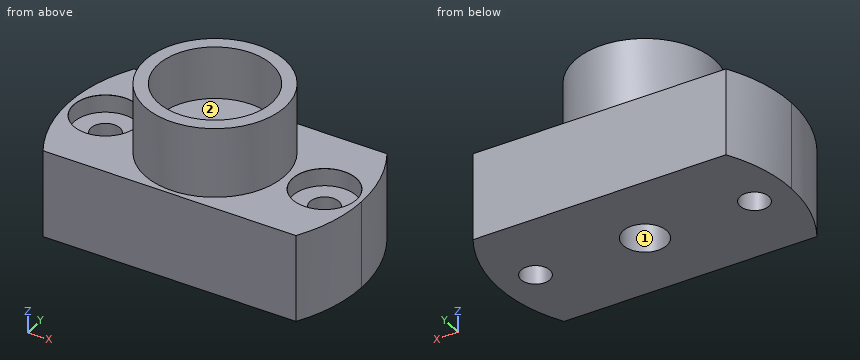
```python
from build123d import *

# Parameters (mm, degrees)
SKETCH1_W                              = 67
SKETCH1_H                              = 34
BOSS_EXTRUDE1_DEPTH                    = 20
CUT_EXTRUDE1_START                     = -20
CUT_EXTRUDE1_DEPTH                     = 20
SKETCH3_R                              = 16
BOSS_EXTRUDE2_DEPTH                    = 16
CBORE_FOR_M6_HEX_HEAD_BOLT1_AT_2_COUNT = 2
CBORE_FOR_M6_HEX_HEAD_BOLT1_AT_2_PITCH = 50
SKETCH9_R                              = 5
CUT_EXTRUDE2_DEPTH                     = 46
SKETCH10_R                             = 13
CUT_EXTRUDE3_DEPTH                     = 12


# Read off the part's stored shape, not the designer's step: Cut-Extrude1
with BuildPart() as part:
    # Sketch1 → Boss-Extrude1 (new body)
    with BuildSketch(Plane.XY):
        Rectangle(SKETCH1_W, SKETCH1_H)
    extrude(amount=BOSS_EXTRUDE1_DEPTH)

    # Cut-Extrude1 outline → Cut-Extrude1 (cut)
    with BuildSketch(Plane.XY.offset(20).offset(CUT_EXTRUDE1_START)):
        with BuildLine():
            ThreePointArc((-33.5, -3.1e-08), (-32.320762268, 8.810126358), (-28.866070048, 17))
            Line((-28.866070048, 17), (-33.5, 17))
            Line((-33.5, 17), (-33.5, -3.1e-08))
        make_face()
        with BuildLine():
            ThreePointArc((-28.866070048, -17), (-32.32076226, -8.810126387), (-33.5, -3.1e-08))
            Line((-33.5, -3.1e-08), (-33.5, -17))
            Line((-33.5, -17), (-28.866070048, -17))
        make_face()
        with BuildLine():
            Line((33.5, 17), (28.866070048, 17))
            ThreePointArc((28.866070048, 17), (32.32076226, 8.810126387), (33.5, 3.1e-08))
            Line((33.5, 3.1e-08), (33.5, 17))
        make_face()
        with BuildLine():
            Line((33.5, -17), (33.5, 3.1e-08))
            ThreePointArc((33.5, 3.1e-08), (32.320762268, -8.810126358), (28.866070048, -17))
            Line((28.866070048, -17), (33.5, -17))
        make_face()
    extrude(amount=CUT_EXTRUDE1_DEPTH, mode=Mode.SUBTRACT)

    # Sketch3 → Boss-Extrude2 (add)
    with BuildSketch(Plane.XY.offset(20)):
        Circle(SKETCH3_R)
    extrude(amount=BOSS_EXTRUDE2_DEPTH)

    # Sketch8 → CBORE for M6 Hex Head Bolt1 (revolve, cut)
    with BuildSketch(Plane(origin=(-25, 0, 20), x_dir=(0, -1, 0), z_dir=(1, 0, 0))):
        Polygon((0, 0), (0, 20), (3.3, 20), (3.3, 4), (7.2735, 4), (7.2735, 0.025), (7.2985, 0), align=None)
    cbore_for_m6_hex_head_bolt1 = revolve(axis=Axis((-25, 0, 26.35), (0, 0, -1)), mode=Mode.SUBTRACT)

    # CBORE for M6 Hex Head Bolt1 at 2: CBORE for M6 Hex Head Bolt1 ×2
    with Locations(*[(i * CBORE_FOR_M6_HEX_HEAD_BOLT1_AT_2_PITCH, 0, 0) for i in range(1, CBORE_FOR_M6_HEX_HEAD_BOLT1_AT_2_COUNT)]):
        add(cbore_for_m6_hex_head_bolt1, mode=Mode.SUBTRACT)

    # Sketch9 → Cut-Extrude2 (cut)
    with BuildSketch(Plane.XY.offset(36)):
        Circle(SKETCH9_R)
    extrude(amount=-CUT_EXTRUDE2_DEPTH, mode=Mode.SUBTRACT)

    # Sketch10 → Cut-Extrude3 (cut)
    with BuildSketch(Plane.XY.offset(36)):
        Circle(SKETCH10_R)
    extrude(amount=-CUT_EXTRUDE3_DEPTH, mode=Mode.SUBTRACT)


solid = part.part
```
Read the model definition and answer for the solid it produces. Units are mm, in the model's axes. Face numbers are marked on the shaded views. A direction names the side the tool comes from. Coordinates: 2 decimals unless noted, no trailing zeros. Write each loop counter-clockwise with the first axis right and the second up, starting at its lowest first coordinate (ties: lowest second). Pieces come first, ordered by that corner, then holes. Notation, with made-up numbers: (15.5, 56) -> (22.5, 56) arc R10 ccw to (22.5, 63) -> close; hole circle Ø5 at (77.25, -2). An arc over 180 degrees is marked (long way). Answer as a JSON object with one key per item and string values.
Q1. Flat-ended cylindrical pins translate along their axes: pin 1 Ø4 at (y, z) = (-11, 28.5) entering from -X; pin 2 Ø1 at (x, z) = (-3, 25.5) entering from -Y; pin 3 Ø4.5 at (x, y) = (-24, 2) entering from +Z. Find the tip coordinate at first contact, or state that the pin passes through.
The answers:
{"pin 1": "stops at x = -13.23", "pin 2": "stops at y = -15.8", "pin 3": "stops at z = 16"}
Q2. The part is cut by section D-D on y = -2. Give the number of separate pieces and of enclosed holes in the cut face, then the cut area to 3 significant figures.
The answers:
{"separate pieces": "4", "enclosed holes": "0", "area": "1,040 mm2"}
Q3. The part is cut by section C-C on x = 0. Give the vertices of the cut face in (y, z).
The answers:
{"outline": "(-17, 0) -> (-5, 0) -> (-5, 24) -> (-13, 24) -> (-13, 36) -> (-16, 36) -> (-16, 20) -> (-17, 20) -> close; (5, 0) -> (17, 0) -> (17, 20) -> (16, 20) -> (16, 36) -> (13, 36) -> (13, 24) -> (5, 24) -> close"}
Q4. A tool of negligible diameter and unlimited length cuts with its end or side. For the marked faces 1 and 2, from which of +Z, -Z, +X, -X, +Y, -Y can it reach the whole face along a straight path? Write none if from no direction.
The answers:
{"face 1": "+Z, -Z", "face 2": "+Z"}
Q5. The part is cut by section B-B on z = 23. Give the vertices of the cut face in (x, y).
The answers:
{"outline": "circle Ø32 at (0, 0); hole circle Ø10 at (0, 0)"}
Q6. Consider line 1 (Y direction, x = -25, z = 6.25); line 2 (Y direction, x = -2, z = 24.5); line 3 (X direction, y = 3, z = 27.5). Determine where each line is inside the solid, lowest interval first. Write a range as [from, to].
The answers:
{"line 1": "y = [-17, -3.3], [3.3, 17]", "line 2": "y = [-15.87, -12.85], [12.85, 15.87]", "line 3": "x = [-15.72, -12.65], [12.65, 15.72]"}
